Read the model definition and answer for the solid it produces. Units are mm, in the model's axes. Coordinates: 2 decimals unless noted, no trailing zeros. Order: outer loops, then holes, each group sorted by start corner. A loop starts at its lowest first (then second) coordinate and runs counter-clockwise, first axis right, second up. Notation, with made-up numbers: M -6.75,69 L 33.25,69 A36 ccw 33.25,103 Z; hole C 76.5,18.5 d5. An arc over 180 degrees is marked long. Put each result on its own line as item: value.
from build123d import *

# Parameters (mm, degrees)
EXTRUDE1_DEPTH     = 3
SKETCH2_R          = 2.75
SKETCH2_R_2        = 1.6
CUT_EXTRUDE1_DEPTH = 3


with BuildPart() as part:
    # Sketch1 → Extrude1 (new body)
    with BuildSketch(Plane.XY):
        Polygon((-21.510078765, 142.709593142), (-21.510078765, -27.502951786), (253.489921235, -27.502951786), (253.489921235, 142.709593142), (233.489921235, 142.709593142), (233.489921235, 112.497048214), (183.489921235, 62.497048214), (183.489921235, 12.497048214), (163.489921235, -7.502951786), (68.489921235, -7.502951786), (48.489921235, 12.497048214), (48.489921235, 62.497048214), (-1.510078765, 112.497048214), (-1.510078765, 142.709593142), align=None)
        with BuildLine():
            Line((-1.510078765, -5.502951786), (-1.510078765, -4.899921406))
            ThreePointArc((-1.510078765, -4.899921406), (-1.35783783, -4.134554541), (-0.924292327, -3.485707844))
            Line((-0.924292327, -3.485707844), (25.075707673, 22.514292156))
            ThreePointArc((25.075707673, 22.514292156), (27.2552881, 22.947837659), (28.489921235, 21.100078594))
            Line((28.489921235, 21.100078594), (28.489921235, 5.041204091))
            ThreePointArc((28.489921235, 5.041204091), (28.64216217, 4.275837226), (29.075707673, 3.626990528))
            Line((29.075707673, 3.626990528), (36.791436425, -4.088738224))
            ThreePointArc((36.791436425, -4.088738224), (37.224981928, -6.268318651), (35.377222863, -7.502951786))
            Line((35.377222863, -7.502951786), (0.489921235, -7.502951786))
            ThreePointArc((0.489921235, -7.502951786), (-0.924292327, -6.917165349), (-1.510078765, -5.502951786))
        make_face(mode=Mode.SUBTRACT)
        with BuildLine():
            Line((1.904134797, 80.798563404), (27.075707673, 55.626990528))
            ThreePointArc((27.075707673, 55.626990528), (27.66149411, 54.212776966), (27.075707673, 52.798563404))
            Line((27.075707673, 52.798563404), (1.904134797, 27.626990528))
            ThreePointArc((1.904134797, 27.626990528), (-0.27544563, 27.193445026), (-1.510078765, 29.041204091))
            Line((-1.510078765, 29.041204091), (-1.510078765, 79.384349841))
            ThreePointArc((-1.510078765, 79.384349841), (-0.27544563, 81.232108906), (1.904134797, 80.798563404))
        make_face(mode=Mode.SUBTRACT)
        with BuildLine():
            Line((233.489921235, 29.041204091), (233.489921235, 79.384349841))
            ThreePointArc((233.489921235, 79.384349841), (232.2552881, 81.232108906), (230.075707673, 80.798563404))
            Line((230.075707673, 80.798563404), (204.904134797, 55.626990528))
            ThreePointArc((204.904134797, 55.626990528), (204.31834836, 54.212776966), (204.904134797, 52.798563404))
            Line((204.904134797, 52.798563404), (230.075707673, 27.626990528))
            ThreePointArc((230.075707673, 27.626990528), (232.2552881, 27.193445026), (233.489921235, 29.041204091))
        make_face(mode=Mode.SUBTRACT)
        with BuildLine():
            Line((232.904134797, -3.485707844), (206.904134797, 22.514292156))
            ThreePointArc((206.904134797, 22.514292156), (204.72455437, 22.947837659), (203.489921235, 21.100078594))
            Line((203.489921235, 21.100078594), (203.489921235, 5.041204091))
            ThreePointArc((203.489921235, 5.041204091), (203.3376803, 4.275837226), (202.904134797, 3.626990528))
            Line((202.904134797, 3.626990528), (195.188406045, -4.088738224))
            ThreePointArc((195.188406045, -4.088738224), (194.754860542, -6.268318651), (196.602619607, -7.502951786))
            Line((196.602619607, -7.502951786), (231.489921235, -7.502951786))
            ThreePointArc((231.489921235, -7.502951786), (232.904134797, -6.917165349), (233.489921235, -5.502951786))
            Line((233.489921235, -5.502951786), (233.489921235, -4.899921406))
            ThreePointArc((233.489921235, -4.899921406), (233.3376803, -4.134554541), (232.904134797, -3.485707844))
        make_face(mode=Mode.SUBTRACT)
    extrude(amount=EXTRUDE1_DEPTH)

    # Sketch2 → Cut-Extrude1 (cut)
    with BuildSketch(Plane.XY.offset(3)):
        with Locations((-14.010076813, 119.997448214)):
            Circle(SKETCH2_R)
        with Locations((-14.010076813, 94.997448214)):
            Circle(SKETCH2_R)
        with Locations((-14.010076813, 34.997448214)):
            Circle(SKETCH2_R)
        with Locations((-14.010076813, 9.997448214)):
            Circle(SKETCH2_R)
        with Locations((-11.510078765, -2.502951786)):
            Circle(SKETCH2_R_2)
        with Locations((-11.510078765, -17.502951786)):
            Circle(SKETCH2_R_2)
        with Locations((8.489921235, -17.502951786)):
            Circle(SKETCH2_R_2)
        with Locations((28.489921235, -17.502951786)):
            Circle(SKETCH2_R_2)
        with Locations((38.489921235, 20.569514271)):
            Circle(SKETCH2_R_2)
        with Locations((38.489921235, 45.569514271)):
            Circle(SKETCH2_R_2)
        with Locations((-11.510078765, 64.709593142)):
            Circle(SKETCH2_R_2)
        with Locations((193.489923187, 45.569514271)):
            Circle(SKETCH2_R_2)
        with Locations((193.489923187, 20.569514271)):
            Circle(SKETCH2_R_2)
        with Locations((203.489923187, -17.502951786)):
            Circle(SKETCH2_R_2)
        with Locations((223.489923187, -17.502951786)):
            Circle(SKETCH2_R_2)
        with Locations((243.489923187, -17.502951786)):
            Circle(SKETCH2_R_2)
        with Locations((245.989921235, 34.997448214)):
            Circle(SKETCH2_R)
        with Locations((245.989921235, 9.997448214)):
            Circle(SKETCH2_R)
        with Locations((243.489923187, 64.709593142)):
            Circle(SKETCH2_R_2)
        with Locations((243.489923187, 134.709593142)):
            Circle(SKETCH2_R_2)
        with Locations((245.989921235, 119.997448214)):
            Circle(SKETCH2_R)
        with Locations((245.989921235, 94.997448214)):
            Circle(SKETCH2_R)
        with Locations((-11.510078765, 134.709593142)):
            Circle(SKETCH2_R_2)
        with Locations((243.489923187, -2.502951786)):
            Circle(SKETCH2_R_2)
    extrude(amount=-CUT_EXTRUDE1_DEPTH, mode=Mode.SUBTRACT)


solid = part.part
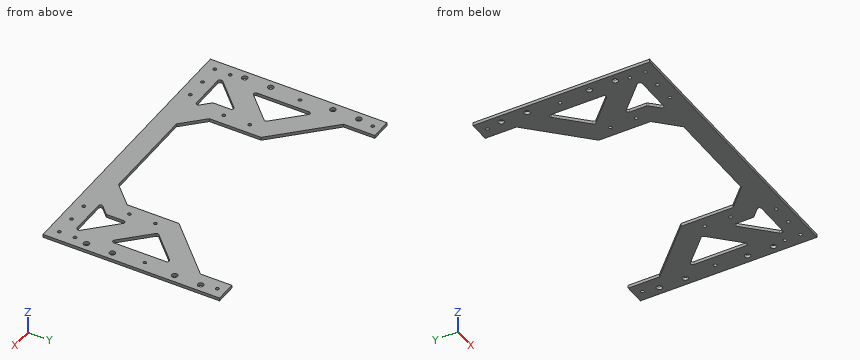
Q1. Find section A-A on y = 86.5. Write down the section's boundary in (x, z), plus the area to 3 significant figures.
Answers below:
outline: M -21.51,0 L 24.49,0 L 24.49,3 L -21.51,3 Z; M 207.49,0 L 253.49,0 L 253.49,3 L 207.49,3 Z
area: 276 mm^2
Q2. Consider line 1 along X through (y, z) = (41.5, 1.15); line 2 along X through (y, z) = (125.5, 2.85); line 3 along X through (y, z) = (13, 0.1). Determine where each line is inside the solid, lowest interval first.
Answers below:
line 1: x = -21.51 to -1.51, 15.78 to 48.49, 183.49 to 216.2, 233.49 to 253.49
line 2: x = -21.51 to -1.51, 233.49 to 253.49
line 3: x = -21.51 to 15.56, 28.49 to 48.49, 183.49 to 203.49, 216.42 to 253.49
Q3. Find section B-B on x = 141. Write down the section's boundary in (y, z), plus the area to 3 significant figures.
Answers below:
outline: M -27.5,0 L -7.5,0 L -7.5,3 L -27.5,3 Z
area: 60.0 mm^2
Q4. Find section C-C on z = 0.65. Give the number of separate pieces and of enclosed holes in the cut face, plus the area to 3 significant figures.
Answers below:
separate pieces: 1
enclosed holes: 28
area: 18,100 mm^2
